Could you check a few things on this drawing? It's one solid part, dimensions in mm from its lowest x, y, z. Coordinates: 2 decimals unless noted, no trailing zeros. Write each loop counter-clockwise with the first axis right and the second up, starting at its lowest first coordinate (ties: lowest second). Pieces come first, ordered by that corner, then holes.
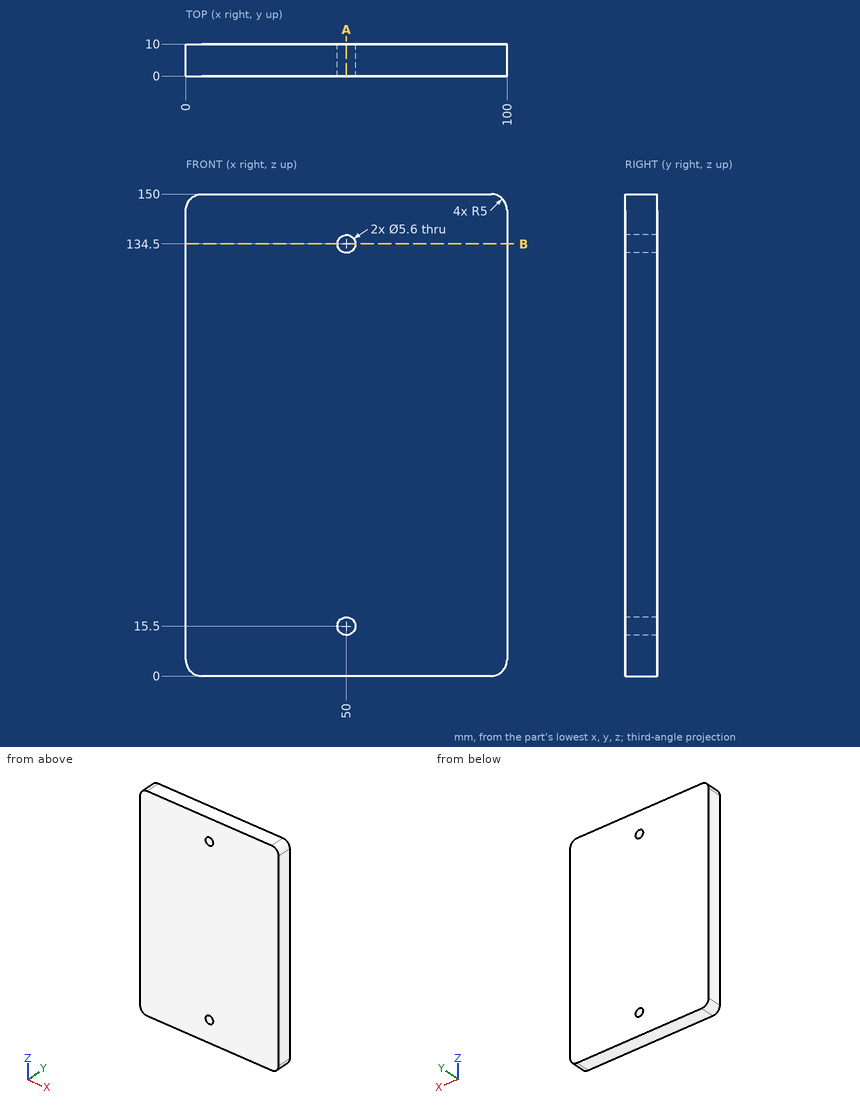
1) I need wall thicknesses on probe 1 along Z at (x, y) = (50, 5); probe 2 along X at (y, z) = (6.25, 134.5); probe 3 along Z at (x, y) = (52, 0.5). Which ranges of each line are inside material? Lowest first, please.
Values follow:
probe 1: z = 0 to 12.7, 18.3 to 131.7, 137.3 to 150
probe 2: x = 0 to 47.2, 52.8 to 100
probe 3: z = 0 to 13.54, 17.46 to 132.54, 136.46 to 150
2) Imagine slicing it at B-B on z = 134.5. Please give me the cut outline in (x, y), then the cut area to 3 significant figures.
Values follow:
outline: (0, 0) - (47.2, 0) - (47.2, 10) - (0, 10) - close; (52.8, 0) - (100, 0) - (100, 10) - (52.8, 10) - close
area: 944 mm2
3) Will this pin go through, and if not, where does the flat tip stop? pin 1 (4 mm diameter, centred on x = 26, y = 7, fed in from -Z).
Values follow:
pin 1: stops at z = 0
4) Imagine slicing it at A-A on x = 50. Please give me the cut outline in (y, z), then the cut area to 3 significant figures.
Values follow:
outline: (0, 0) - (10, 0) - (10, 12.7) - (0, 12.7) - close; (0, 18.3) - (10, 18.3) - (10, 131.7) - (0, 131.7) - close; (0, 137.3) - (10, 137.3) - (10, 150) - (0, 150) - close
area: 1,390 mm2
